from build123d import *

# Parameters (mm, degrees)
F0_R     = 50.8
F1_DEPTH = 76.2
F1_TAPER = 8
F2_W     = 127
F2_H     = 15.875
F3_DEPTH = 20.32
F4_R     = 48.30064
F5_DEPTH = 49.276
F5_TAPER = 8


with BuildPart() as f1:
    # F0 (on Top) → F1 (new body)
    with BuildSketch(Plane.XY):
        Circle(F0_R)
    extrude(amount=F1_DEPTH, taper=F1_TAPER)

    # F2 (on face) → F3 (cut)
    with BuildSketch(Plane.XY.offset(76.2)):
        Rectangle(F2_W, F2_H)
    extrude(amount=-F3_DEPTH, mode=Mode.SUBTRACT)

    # F4 (on face) → F5 (cut)
    with BuildSketch(Plane(origin=(0, 0, 0), x_dir=(1, 0, 0), z_dir=(0, 0, -1))):
        Circle(F4_R)
    extrude(amount=-F5_DEPTH, taper=F5_TAPER, mode=Mode.SUBTRACT)


solid = f1.part
Could you check a few things on this model? Use its own coordinates, in mm. A direction names the side the tool comes from. Give positions to 0.01 mm unless a question says otherwise; leave off trailing zeros. Order: outer loops, then holes, each group sorted by start corner. A loop starts at its lowest first (then second) coordinate and runs counter-clockwise, first axis right, second up. Notation, with made-up numbers: (64.25, -18) -> (70.25, -18) arc R21 ccw to (70.25, 21) -> close; hole circle Ø3 at (35, 31.5). An arc over 180 degrees is marked (long way). Answer in a Markdown table with one row per item. Add a question column.
Item 1: We'd pull the mould along Y, two halves only. Please class faces 3 (the flat face through (-1, -1, 49.276)), 4 (the conical face through (40.81, -16.92, 47.1)), 5 (the flat face through (-1, -20, 76.2)): pulls with the +Y half, pulls with the -Y half, needs draft (parallel to the pull), parting line crosses it, or undercut.
Item 2: Imagine slicing it at D-D (z = 7.5). List the corners of the cut face in (x, y) for me.
Item 3: Please list where these lines run through material, in increasing order: probe 1 along Z at (x, y) = (25, 10); probe 2 along Y at (x, z) = (18.5, 63); probe 3 along X at (y, z) = (38, 32.5).
Item 4: For faces 1 (the flat face through (-1, 21, 76.2)), 2 (the flat face through (-1, 7.938, 66)), which set-ups out of +Z, -Z, +X, -X, +Y, -Y let a thin tool reach every point of the face, with its end or its side?
Item 5: Imagine slicing it at C-C (z = 47). List the corners of the cut face in (x, y) for me.
Item 6: Imagine slicing it at B-B (z = 65). List the corners of the cut face in (x, y) for me.
Item 7: Imagine slicing it at A-A (x = 0). List the corners of the cut face in (y, z) for me.
Item 8: I'm going to push flat-ended pins straight in: P1, Ø2, axis at x = 9.5, z = 58.5, coming from the -Y side; P2, Ø25, axis at x = 20.5, y = -17, coming from the -Z side; P3, Ø4, axis at x = -19.5, z = 65.5, coming from the +Y side. Where does each tip first touch, or does it pass through?
Result:
| question | item | result |
|---|---|---|
| 1 | face 3 | undercut |
| 1 | face 4 | parting line crosses it |
| 1 | face 5 | needs draft |
| 2 | outline | circle Ø99.49 at (0, 0); hole circle Ø94.49 at (0, 0) |
| 3 | probe 1 | 49.28 to 76.2 |
| 3 | probe 2 | -37.65 to -7.94, 7.94 to 37.65 |
| 3 | probe 3 | -26.33 to -21.65, 21.65 to 26.33 |
| 4 | face 1 | +Z, +X, -X, +Y, -Y |
| 4 | face 2 | +Z, +X, -X |
| 5 | outline | circle Ø88.39 at (0, 0); hole circle Ø83.39 at (0, 0) |
| 6 | outline | (-40.9, -7.94) arc R41.66 ccw to (40.9, -7.94) -> close; (-40.9, 7.94) -> (40.9, 7.94) arc R41.66 ccw to start |
| 7 | outline | (-50.8, 0) -> (-48.3, 0) -> (-41.38, 49.28) -> (41.38, 49.28) -> (48.3, 0) -> (50.8, 0) -> (40.09, 76.2) -> (7.94, 76.2) -> (7.94, 55.88) -> (-7.94, 55.88) -> (-7.94, 76.2) -> (-40.09, 76.2) -> close |
| 8 | P1 | y = -41.77 |
| 8 | P2 | z = 49.28 |
| 8 | P3 | y = 37.78 |
